The model under review builds one solid part; all positions refer to its coordinate system, in mm. Face numbers are marked on the shaded views. A direction names the side the tool comes from. Round coordinates to 2 decimals unless told otherwise and drop trailing zeros. Loops run counter-clockwise (first coordinate to the right, second up) from the corner with the lowest first, then second, coordinate; pieces in that order, holes last. Notation, with made-up numbers: M -33.75,-13 L 11.25,-13 A19 ccw 11.25,22 Z; hole C 18.25,68 d5. An arc over 180 degrees is marked long. Answer in a Markdown table with one row per item. Add a question column.
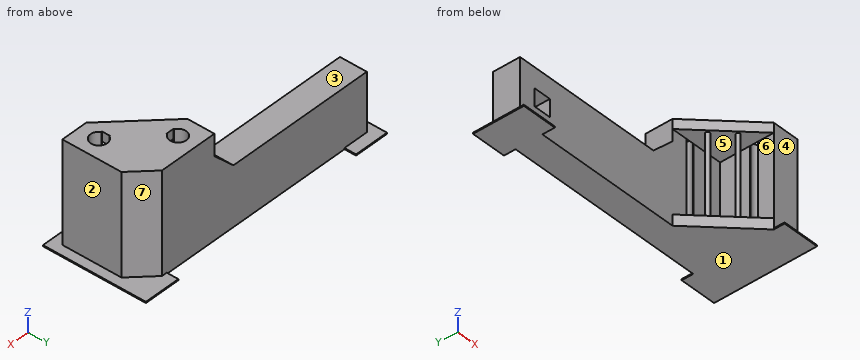
from build123d import *

# Parameters (mm, degrees)
PAD_DEPTH     = 17
PAD001_DEPTH  = 2
PAD002_DEPTH  = 1.8
SKETCH003_W   = 32
SKETCH003_H   = 11
PAD003_DEPTH  = 5
SKETCH004_W   = 3.25
SKETCH004_H   = 3.25
POCKET_DEPTH  = 3.1
SKETCH005_W   = 6.497684
SKETCH005_H   = 9.461539
SKETCH005_W_2 = 6.809606
SKETCH005_H_2 = 19.151065
PAD004_DEPTH  = 0.225
CHAMFER_SIZE  = 4
SKETCH006_R   = 0.375
PAD005_DEPTH  = 16


with BuildPart() as part:
    # Sketch → Pad (new body)
    with BuildSketch(Plane.XY):
        with BuildLine():
            Line((-10, 0), (-10, 5))
            Line((-10, 5), (5, 5))
            Line((5, 5), (5, -10))
            Line((5, -10), (0, -10))
            Line((0, -7.05), (0, -10))
            Line((0, -7.05), (0.143534, -7.05))
            ThreePointArc((0.143534, -7.05), (3.05, -6.3), (0.143534, -5.55))
            Line((0, -5.55), (0.143534, -5.55))
            Line((0, 0), (0, -5.55))
            Line((0, 0), (-5.55, 0))
            Line((-5.55, 0), (-5.55, 0.143534))
            ThreePointArc((-5.55, 0.143534), (-6.3, 3.05), (-7.05, 0.143534))
            Line((-7.05, 0), (-7.05, 0.143534))
            Line((-10, 0), (-7.05, 0))
        make_face()
    extrude(amount=-PAD_DEPTH)

    # Sketch001 (on Face16 of Pad) → Pad001 (join)
    with BuildSketch(Plane(origin=(0, 0, -17), x_dir=(1, 0, 0), z_dir=(0, 0, -1))):
        Polygon((5, -5), (-10, -5), (-10, 0), (0, 10), (5, 10), align=None)
    extrude(amount=PAD001_DEPTH)

    # Sketch002 (on Face1 of Pad001) → Pad002 (join)
    with BuildSketch(Plane.XY):
        Polygon((0, -10), (0, 0), (-10, 0), align=None)
    extrude(amount=-PAD002_DEPTH)

    # Sketch003 (on Face10 of Pad002) → Pad003 (join)
    with BuildSketch(Plane.XZ):
        with Locations((-26, -13.5)):
            Rectangle(SKETCH003_W, SKETCH003_H)
    extrude(amount=-PAD003_DEPTH)

    # Sketch004 (on Face22 of Pad003) → Pocket (cut)
    with BuildSketch(Plane.XZ):
        with Locations((-37.375, -13.375)):
            Rectangle(SKETCH004_W, SKETCH004_H)
    extrude(amount=-POCKET_DEPTH, mode=Mode.SUBTRACT)

    # Sketch005 → Pad004 (join)
    with BuildSketch(Plane(origin=(0, 0, -19), x_dir=(1, 0, 0), z_dir=(0, 0, -1))):
        with Locations((-40.563391, -2.425933)):
            Rectangle(SKETCH005_W, SKETCH005_H)
        with Locations((3.404803, 2.422745)):
            Rectangle(SKETCH005_W_2, SKETCH005_H_2)
    extrude(amount=-PAD004_DEPTH)

    # Chamfer
    chamfer_edges = [part.edges().sort_by_distance(p)[0] for p in [
        (-10, 2.5, -8),
        (5, 5, -9.3875),
    ]]
    chamfer(chamfer_edges, length=CHAMFER_SIZE)

    # Sketch006 (on Face29 of Chamfer) → Pad005 (join)
    with BuildSketch(Plane.XY.offset(-17)):
        with Locations((-6, -3)):
            Circle(SKETCH006_R)
        with Locations((-3, -6)):
            Circle(SKETCH006_R)
    extrude(amount=PAD005_DEPTH)


solid = part.part
1. Mouldability with a two-part tool opening along X and no side actions: class the marked faces 4, 5, 6 and 7 as released by +X, released by -X, zero draft, split by the parting line, or undercut.
2. Take a section at A-A, the plane z = -5. State the section outline as (x, y) points (3 decimals).
3. Take a section at D-D, the plane z = -7.5. State the section outline as (x, y) points (3 decimals), and give its area (3 significant figures).
4. To check wall thickness, follow probe 1 along Z at (x, y) = (-14, 0.25); probe 2 along X at (y, z) = (-0.5, -10); probe 3 along Y at (x, z) = (1.5, -4.5). State the ranges of each line that lie inside material, in increasing order.
5. Take a section at C-C, the plane x = 1.5. State the section outline as (y, z) points (3 decimals), and give its area (3 significant figures).
6. Machinability: for the marked faces 1, 2 and 3, which of the approach directions +Z, -Z, +X, -X, +Y, -Y give a long, thin tool a straight path to every point of the face, cutting with its end or side? Answer none if there is none.
7. For pin 1 Ø1.6 at (x, y) = (-38, 1.5) entering from +Z; pin 2 Ø8 at (y, z) = (-9.5, -12.5) entering from -X (3 decimals); pin 3 Ø1.5 at (y, z) = (2.5, -15) entering from -X, all flat-tipped, find the tip position at first contact; note any pin that passes through.
8. Take a section at B-B, the plane z = -1.25. State the section outline as (x, y) points, and give its area (3 significant figures).
Check sheet entries:
| question | item | result |
|---|---|---|
| 1 | face 4 | zero draft |
| 1 | face 5 | undercut |
| 1 | face 6 | released by -X |
| 1 | face 7 | released by +X |
| 2 | outline | M -11,0 L -7.05,0 L -7.05,0.144 A1.55 cw long -5.55,0.144 L -5.55,0 L 0,0 L 0,-5.55 L 0.144,-5.55 A1.55 cw long 0.144,-7.05 L 0,-7.05 L 0,-10 L 5,-10 L 5,1 L 1,5 L -11,5 Z; C -6,-3 d0.75; C -3,-6 d0.75 |
| 3 | outline | M -13.5,0 L -7.05,0 L -7.05,0.144 A1.55 cw long -5.55,0.144 L -5.55,0 L 0,0 L 0,-5.55 L 0.144,-5.55 A1.55 cw long 0.144,-7.05 L 0,-7.05 L 0,-10 L 5,-10 L 5,1 L 1,5 L -13.5,5 Z; C -6,-3 d0.75; C -3,-6 d0.75 |
| 3 | area | 120 mm^2 |
| 4 | probe 1 | z = -19 to -8 |
| 4 | probe 2 | x = 0 to 5 |
| 4 | probe 3 | y = -10 to -7.85, -4.75 to 4.5 |
| 5 | outline | M -11.998,-19 L 7.153,-19 L 7.153,-18.775 L 4.5,-18.775 L 4.5,0 L -4.75,0 L -4.75,-17 L -7.85,-17 L -7.85,0 L -10,0 L -10,-18.775 L -11.998,-18.775 Z |
| 5 | area | 224 mm^2 |
| 6 | face 1 | -Z, +X, -X, +Y, -Y |
| 6 | face 2 | +Z, +X, +Y, -Y |
| 6 | face 3 | +Z, -X, +Y, -Y |
| 7 | pin 1 | stops at z = -8 |
| 7 | pin 2 | stops at x = -3.375 |
| 7 | pin 3 | stops at x = -42 |
| 8 | outline | M -10,0 L 0,-10 L 5,-10 L 5,1 L 1,5 L -10,5 Z; hole M -7.05,0 L -5.55,0 L -5.55,0.14 A1.55 ccw long -7.05,0.14 Z; hole M 0,-7.05 L 0.14,-7.05 A1.55 ccw long 0.14,-5.55 L 0,-5.55 Z |
| 8 | area | 152 mm^2 |
